Geometry check sheet. Reference: the model listing, model coordinates, mm. A direction names the side the tool comes from. Give positions to 0.01 mm unless a question says otherwise; leave off trailing zeros. Order: outer loops, then holes, each group sorted by start corner. A loop starts at its lowest first (then second) coordinate and runs counter-clockwise, first axis right, second up. Notation, with made-up numbers: M 30,27 L 60,27 A24 cw 60,46 Z; hole C -7,53 d2. An arc over 180 degrees is marked long. One line per question, with ' | ' between items. Start each with the question number.
from build123d import *

# Parameters (mm, degrees)
F0_W     = 50
F0_H     = 32
F0_R     = 1.6
F1_DEPTH = 6
F2_R     = 3
F3_DEPTH = 3
F4_R     = 2.6
F5_DEPTH = 25.4
F6_R     = 11
F7_DEPTH = 25.4
F8_R     = 6


with BuildPart() as f1:
    # F0 (on Top) → F1 (new body)
    with BuildSketch(Plane.XY):
        Rectangle(F0_W, F0_H)
        with Locations((-10.3261368227, -10)):
            Circle(F0_R, mode=Mode.SUBTRACT)
        with Locations((9.6738631773, -9.6330129863)):
            Circle(F0_R, mode=Mode.SUBTRACT)
        with Locations((-10, 10)):
            Circle(F0_R, mode=Mode.SUBTRACT)
        with Locations((10, 10.3669870137)):
            Circle(F0_R, mode=Mode.SUBTRACT)
    extrude(amount=F1_DEPTH)

    # F2 (on face) → F3 (cut)
    with BuildSketch(Plane.XY.offset(6)):
        with Locations((-10, 10)):
            Circle(F2_R)
        with Locations((-10.3261368227, -10)):
            Circle(F2_R)
        with Locations((9.6738631773, -9.6330129863)):
            Circle(F2_R)
        with Locations((10, 10.3669870137)):
            Circle(F2_R)
    extrude(amount=-F3_DEPTH, mode=Mode.SUBTRACT)

    # F4 (on face) → F5 (cut)
    with BuildSketch(Plane.XY.offset(6)):
        with Locations((-20, 0)):
            Circle(F4_R)
        with Locations((20, 0)):
            Circle(F4_R)
    extrude(amount=-F5_DEPTH, mode=Mode.SUBTRACT)

    # F6 (on face) → F7 (cut)
    with BuildSketch(Plane.XY.offset(6)):
        with Locations((-25, 16)):
            Circle(F6_R)
        with Locations((25, 16)):
            Circle(F6_R)
        with Locations((25, -16)):
            Circle(F6_R)
        with Locations((-25, -16)):
            Circle(F6_R)
    extrude(amount=-F7_DEPTH, mode=Mode.SUBTRACT)

    # F8
    f8_edges = [f1.edges().sort_by_distance(p)[0] for p in [
        (-14, -16, 3),
        (-25, -5, 3),
        (14, -16, 3),
        (25, -5, 3),
        (25, 5, 3),
        (14, 16, 3),
        (-14, 16, 3),
        (-25, 5, 3),
    ]]
    fillet(f8_edges, radius=F8_R)


solid = f1.part
Item 1: Cross-section at B-B, the plane z = 1.05. Record the cut outline in (x, y).
Item 2: Cross-section at C-C, the plane x = -10. Record the cut outline in (y, z).
Item 3: Cross-section at A-A, the plane x = 20. Record the cut outline in (y, z), plus the area to 3 significant figures.
Item 4: Cross-section at D-D, the plane z = 4.55. Record the cut outline in (x, y), plus the area to 3 significant figures.
Item 5: Mould release check, pull along Y, two halves, no side actions. Record for faces 3 (the cylindrical face through (23.906, 3.548, 3.042)), 4 (the cylindrical face through (-12.548, -14.906, 2.958)), 5 (the flat face through (-8.7, 8.7, 3)), 6 (the flat face through (11, -11, 3)): released by +Y, released by -Y, zero draft, split by the parting line, or undercut.
Item 6: Depth check by flat-ended pin: pin 1 (4 mm diameter, centred on x = -10.33, y = -10, fed in from +Z); pin 2 (1 mm diameter, centred on x = -16, z = 4.5, fed in from +Y). Enter the tip coordinate at first touch or a pass-through.
Item 7: Set-up check for faces 1 (the cylindrical face through (-17.176, -8.268, 3.042)), 2 (the cylindrical face through (-12.4, 8.2, 4.5)): record each of +Z, -Z, +X, -X, +Y, -Y from which the full face is reachable in a straight line by a thin tool's end or side.
Item 8: Material ranges on line 1 along Y through (x, z) = (-9, 0.5); line 2 along X through (y, z) = (1, 0.3); line 3 along X through (y, z) = (-12, 4.05), recorded low to high.
Outcome:
1) outline: M -25,-0.09 A6 ccw -21.12,-5.71 A11 cw -14.71,-12.12 A6 ccw -9.09,-16 L 9.09,-16 A6 ccw 14.71,-12.12 A11 cw 21.12,-5.71 A6 ccw 25,-0.09 L 25,0.09 A6 ccw 21.12,5.71 A11 cw 14.71,12.12 A6 ccw 9.09,16 L -9.09,16 A6 ccw -14.71,12.12 A11 cw -21.12,5.71 A6 ccw -25,0.09 Z; hole C -20,0 d5.2; hole C -10.33,-10 d3.2; hole C -10,10 d3.2; hole C 9.67,-9.63 d3.2; hole C 10,10.37 d3.2; hole C 20,0 d5.2
2) outline: M -15.93,0 L -11.57,0 L -11.57,3 L -12.98,3 L -12.98,6 L -15.93,6 Z; M -8.43,0 L 8.4,0 L 8.4,3 L 7,3 L 7,6 L -7.02,6 L -7.02,3 L -8.43,3 Z; M 11.6,0 L 15.93,0 L 15.93,6 L 13,6 L 13,3 L 11.6,3 Z
3) outline: M -6.2,0 L -2.6,0 L -2.6,6 L -6.2,6 Z; M 2.6,0 L 6.2,0 L 6.2,6 L 2.6,6 Z | area: 43.2 mm²
4) outline: M -25,-0.09 A6 ccw -21.12,-5.71 A11 cw -14.71,-12.12 A6 ccw -9.09,-16 L 9.09,-16 A6 ccw 14.71,-12.12 A11 cw 21.12,-5.71 A6 ccw 25,-0.09 L 25,0.09 A6 ccw 21.12,5.71 A11 cw 14.71,12.12 A6 ccw 9.09,16 L -9.09,16 A6 ccw -14.71,12.12 A11 cw -21.12,5.71 A6 ccw -25,0.09 Z; hole C -20,0 d5.2; hole C -10.33,-10 d6; hole C -10,10 d6; hole C 9.67,-9.63 d6; hole C 10,10.37 d6; hole C 20,0 d5.2 | area: 1,030 mm²
5) face 3: released by +Y | face 4: released by -Y | face 5: undercut | face 6: undercut
6) pin 1: stops at z = 3 | pin 2: stops at y = 10.45
7) face 1: +Z, -Z, -X, -Y | face 2: +Z
8) line 1: y = -16 to -10.9, -9.1 to 8.75, 11.25 to 16 | line 2: x = -24.93 to -22.4, -17.6 to 17.6, 22.4 to 24.93 | line 3: x = -14.75 to -12.56, -8.09 to 7.83, 11.52 to 14.75
